```python
from build123d import *

# Parameters (mm, degrees)
SKETCH1_W           = 46
SKETCH1_H           = 73
BOSS_EXTRUDE1_DEPTH = 2
SKETCH2_W           = 2
SKETCH2_H           = 5
BOSS_EXTRUDE2_DEPTH = 3
BOSS_EXTRUDE3_DEPTH = 5
FILLET1_R           = 0.6
FILLET2_R           = 5
SKETCH5_W           = 46
SKETCH5_H           = 73
SKETCH5_W_2         = 42
SKETCH5_H_2         = 69
CUT_EXTRUDE1_DEPTH  = 10
FILLET3_R           = 1
SKETCH6_W           = 4.312342675
SKETCH6_H           = 2.937978419
SKETCH6_W_2         = 4.686780993
SKETCH6_H_2         = 2.65792504
CUT_EXTRUDE2_DEPTH  = 10
BOSS_EXTRUDE4_DEPTH = 5
FILLET4_R           = 0.6


with BuildPart() as part:
    # Sketch1 → Boss-Extrude1 (new body)
    with BuildSketch(Plane.XY):
        with Locations((23, -36.5)):
            Rectangle(SKETCH1_W, SKETCH1_H)
    extrude(amount=BOSS_EXTRUDE1_DEPTH)

    # Sketch2 → Boss-Extrude2 (add)
    with BuildSketch(Plane.XY.offset(2)):
        with Locations((3, -37)):
            Rectangle(SKETCH2_W, SKETCH2_H)
        with Locations((43, -37)):
            Rectangle(SKETCH2_W, SKETCH2_H)
    extrude(amount=BOSS_EXTRUDE2_DEPTH)

    # Sketch3 → Boss-Extrude3 (add)
    with BuildSketch(Plane.XZ.offset(39.5)):
        Polygon((2, 5), (0, 5), (2, 7), (4, 7), (4, 5), align=None)
        Polygon((44, 5), (46, 5), (44, 7), (42, 7), (42, 5), align=None)
    extrude(amount=-BOSS_EXTRUDE3_DEPTH)

    # Fillet1
    fillet1_edges = [part.edges().sort_by_distance(p)[0] for p in [
        (0, -37, 5),
        (46, -37, 5),
    ]]
    fillet(fillet1_edges, radius=FILLET1_R)

    # Fillet2
    fillet2_edges = [part.edges().sort_by_distance(p)[0] for p in [
        (0, 0, 1),
        (46, 0, 1),
    ]]
    fillet(fillet2_edges, radius=FILLET2_R)

    # Sketch5 → Cut-Extrude1 (cut)
    with BuildSketch(Plane.XY.offset(2)):
        with Locations((23, -36.5)):
            Rectangle(SKETCH5_W, SKETCH5_H)
        with Locations((23, -36.5)):
            Rectangle(SKETCH5_W_2, SKETCH5_H_2, mode=Mode.SUBTRACT)
    extrude(amount=-CUT_EXTRUDE1_DEPTH, mode=Mode.SUBTRACT)

    # Fillet3
    fillet3_edges = [part.edges().sort_by_distance(p)[0] for p in [
        (2, -2, 1),
        (44, -2, 1),
    ]]
    fillet(fillet3_edges, radius=FILLET3_R)

    # Sketch6 → Cut-Extrude2 (cut)
    with BuildSketch(Plane.XZ.offset(39.5)):
        with Locations((1.843828662, 6.46898921)):
            Rectangle(SKETCH6_W, SKETCH6_H)
        with Locations((44.343390497, 6.32896252)):
            Rectangle(SKETCH6_W_2, SKETCH6_H_2)
    extrude(amount=-CUT_EXTRUDE2_DEPTH, mode=Mode.SUBTRACT)

    # Sketch7 → Boss-Extrude4 (add)
    with BuildSketch(Plane.XZ.offset(39.5)):
        Polygon((2, 2.5), (0, 2.5), (2, 5), (4, 5), (4, 2.5), align=None)
        Polygon((42, 2.5), (46, 2.5), (44, 5), (42, 5), align=None)
    extrude(amount=-BOSS_EXTRUDE4_DEPTH)

    # Fillet4
    fillet4_edges = [part.edges().sort_by_distance(p)[0] for p in [
        (0, -37, 2.5),
        (46, -37, 2.5),
    ]]
    fillet(fillet4_edges, radius=FILLET4_R)


solid = part.part
```
Input: part model. Units: mm. Frame: model coordinates. A direction names the side the tool comes from. Give positions to 0.01 mm unless a question says otherwise; leave off trailing zeros. Loops run counter-clockwise (first coordinate to the right, second up) from the corner with the lowest first, then second, coordinate; pieces in that order, holes last. Notation, with made-up numbers: M -23.75,40 L 15.25,40 A19 cw 15.25,56 Z; hole C 62.25,75 d9. An arc over 180 degrees is marked long. Answer as CSV lines item,"result". Start each with the question number.
1. Section C-C on x = 8.5. Return loops of the section in (y, z), plus the area to 3 significant figures.
2. Reachability of faces 5 (the face through (3, -39.5, 4)), 6 (the face through (43, -34.5, 3)), 7 (the face through (2, -37, 1)), 8 (the face through (44, -37, 1)), 9 (the face through (4, -37, 4)) from +Z, -Z, +X, -X, +Y, -Y: full face, straight path, thin tool, end or side. Return the list, or none.
3. Section B-B on y = -6.5. Return loops of the section in (x, z), plus the area to 3 significant figures.
4. Section A-A on z = 4.3. Return loops of the section in (x, y), plus the area to 3 significant figures.
5. Section D-D on z = 1.05. Return loops of the section in (x, y).
6. Pull-direction query (X, two-part tool) for faces 1 (the face through (44.619, -37.035, 4.227)), 2 (the face through (1.381, -37.035, 4.227)), 3 (the face through (3, -34.5, 4)), 4 (the face through (42, -37, 3)); classes: released by +X, released by -X, zero draft, split by the parting line, or undercut.
7. Line query: L1, parallel to X at y = -14, z = 1.3; L2, parallel to Z at x = 4.5, y = -6.5; L3, parallel to Y at x = 42.5, z = 4.65. Output: solid intervals per line, ascending.
8. Pin query (flat end, axial travel): P1, Ø0.8, axis at y = -37.5, z = 2, coming from the +X side; P2, Ø6, axis at x = 14, y = -58.5, coming from the +Z side; P3, Ø2.5, axis at x = 44.5, z = 4, coming from the +Y side. Return the tip coordinate at first contact, or that it passes through.
Computed values:
1,outline,"M -71,0 L -2,0 L -2,2 L -71,2 Z"
1,area,"138 mm²"
2,face 5,"+Z, +X, -X, -Y"
2,face 6,"+Z, +X, -X, +Y"
2,face 7,"-Z, -X, +Y, -Y"
2,face 8,"-Z, +X, +Y, -Y"
2,face 9,"+Z, +Y, -Y"
3,outline,"M 2,0 L 44,0 L 44,2 L 2,2 Z"
3,area,"84.0 mm²"
4,outline,"M 1.44,-39.5 L 4,-39.5 L 4,-34.5 L 1.44,-34.5 Z; M 42,-39.5 L 44.56,-39.5 L 44.56,-34.5 L 42,-34.5 Z"
4,area,"25.6 mm²"
5,outline,"M 2,-71 L 44,-71 L 44,-3 A1 ccw 43,-2 L 3,-2 A1 ccw 2,-3 Z"
6,face 1,"released by +X"
6,face 2,"released by -X"
6,face 3,"zero draft"
6,face 4,"undercut"
7,L1,"x = 2 to 44"
7,L2,"z = 0 to 2"
7,L3,"y = -39.5 to -34.5"
8,P1,"stops at x = 44"
8,P2,"stops at z = 2"
8,P3,"stops at y = -34.5"
